```python
from build123d import *

# Parameters (mm, degrees)
F0_W     = 1905
F0_H     = 965.2
F1_DEPTH = 203.2
F2_R     = 127
F3_R     = 12.7


with BuildPart() as f1:
    # F0 (on Top) → F1 (new body)
    with BuildSketch(Plane.XY):
        Rectangle(F0_W, F0_H)
    extrude(amount=F1_DEPTH)

    # F2
    f2_edges = [f1.edges().sort_by_distance(p)[0] for p in [
        (952.5, -482.6, 101.6),
        (-952.5, -482.6, 101.6),
        (952.5, 482.6, 101.6),
        (-952.5, 482.6, 101.6),
    ]]
    fillet(f2_edges, radius=F2_R)

    # F3
    f3_edges = [f1.edges().sort_by_distance(p)[0] for p in [
        (952.5, 0, 203.2),
        (915.302561, -445.402561, 203.2),
        (915.302561, 445.402561, 203.2),
        (0, -482.6, 203.2),
        (0, 482.6, 203.2),
        (-915.302561, -445.402561, 203.2),
        (-915.302561, 445.402561, 203.2),
        (-952.5, 0, 203.2),
        (952.5, 0, 0),
        (915.302561, -445.402561, 0),
        (915.302561, 445.402561, 0),
        (0, -482.6, 0),
        (0, 482.6, 0),
        (-915.302561, -445.402561, 0),
        (-915.302561, 445.402561, 0),
        (-952.5, 0, 0),
    ]]
    fillet(f3_edges, radius=F3_R)

    # F7: sweep along a path in F7_path
    with BuildLine(Plane(origin=(-825.5, -482.6, 190.5), x_dir=(0, 1, 0), z_dir=(0, 0, 1))) as f7_path:
        Line((0, 0), (0, -1651))
        ThreePointArc((0, -1651), (37.1974387893, -1740.8025612107), (127, -1778))
        Line((127, -1778), (838.2, -1778))
        ThreePointArc((838.2, -1778), (928.0025612107, -1740.8025612107), (965.2, -1651))
        Line((965.2, -1651), (965.2, 0))
        ThreePointArc((965.2, 0), (928.0025612107, 89.8025612107), (838.2, 127))
        Line((838.2, 127), (127, 127))
        ThreePointArc((127, 127), (37.1974387893, 89.8025612107), (0, 0))
    # F5 (on face) → F7 (sweep, cut)
    with BuildSketch(Plane.YZ.offset(825.5)):
        with BuildLine():
            Line((-480.06, 21.058702955), (-480.06, 182.141297045))
            ThreePointArc((-480.06, 182.141297045), (-481.7282889113, 186.4312948633), (-485.8565610336, 188.4671333779))
            Line((-485.8565610336, 188.4671333779), (-553.3473393859, 194.3718113762))
            Line((-553.3473393859, 194.3718113762), (-553.3473393859, 8.8281886238))
            Line((-553.3473393859, 8.8281886238), (-485.8565610336, 14.7328666221))
            ThreePointArc((-485.8565610336, 14.7328666221), (-481.7282889113, 16.7687051367), (-480.06, 21.058702955))
        make_face()
    sweep(path=f7_path.line, mode=Mode.SUBTRACT)


solid = f1.part
```
The model under review builds one solid part; all positions refer to its coordinate system, in mm. A direction names the side the tool comes from. Round coordinates to 2 decimals unless told otherwise and drop trailing zeros. Order: outer loops, then holes, each group sorted by start corner. A loop starts at its lowest first (then second) coordinate and runs counter-clockwise, first axis right, second up.
(1) For P1, Ø3, axis at x = 442.5, z = 73.5, coming from the +Y side; P2, Ø10, axis at y = 9, z = 155, coming from the -X side; P3, Ø8, axis at x = 170, z = 142, coming from the -Y side, all flat-tipped, find the tip position at first contact; note any pin that passes through.
Working result:
P1: stops at y = 480.06
P2: stops at x = -949.96
P3: stops at y = -480.06
(2) Mouldability with a two-part tool opening along Z and no side actions: class faces 1 (the face through (949.96, 5, 100)), 2 (the face through (-13, 7, 0)), 3 (the face through (-13, 7, 203.2)), 4 (the face through (-914.5, -442.6, 102.7)) as released by +Z, released by -Z, zero draft, split by the parting line, or undercut.
Working result:
face 1: undercut
face 2: released by -Z
face 3: released by +Z
face 4: undercut
(3) Take a section at A-A, the plane z = 100. State the section outline as (x, y) points, plus the area to 3 significant figures.
Working result:
outline: (-949.96, -355.6) arc R124.46 ccw to (-825.5, -480.06) - (825.5, -480.06) arc R124.46 ccw to (949.96, -355.6) - (949.96, 355.6) arc R124.46 ccw to (825.5, 480.06) - (-825.5, 480.06) arc R124.46 ccw to (-949.96, 355.6) - close
area: 1,810,000 mm2
(4) Tool access review of faces 5 (the face through (914.5, 442.6, 102.7)), 6 (the face through (-949.96, -5, 100)), 7 (the face through (-912.5, 444.6, 102.7)), 8 (the face through (12, -480.06, 100)), 9 (the face through (912.5, -444.6, 102.7)): name each direction out of +Z, -Z, +X, -X, +Y, -Y from which nothing blocks a thin tool from reaching the whole face with its end or side.
Working result:
face 5: +X, +Y
face 6: -X, +Y, -Y
face 7: -X, +Y
face 8: +X, -X, -Y
face 9: +X, -Y
(5) Wall thickness on L1, parallel to X at y = -82.5, z = 169; L2, parallel to Y at x = 517, z = 184; L3, parallel to Y at x = -612, z = 131.5: over which ranges is each line inside the solid? List them lowest first.
Working result:
L1: x = -949.96 to 949.96
L2: y = -480.34 to 480.34
L3: y = -480.06 to 480.06
